```python
from build123d import *

# Parameters (mm, degrees)
BOSS_EXTRUDE1_DEPTH = 40
BOSS_EXTRUDE2_START = -10
SKETCH2_W           = 20
SKETCH2_H           = 50
BOSS_EXTRUDE2_DEPTH = 20
FILLET1_R           = 5
FILLET2_R           = 2
SKETCH3_W           = 45
SKETCH3_H           = 40
BOSS_EXTRUDE3_DEPTH = 5
FILLET3_R           = 5
SKETCH4_R           = 1.55
CUT_EXTRUDE1_DEPTH  = 5
MIRROR4_START       = 60
MIRROR4_OUTLINE_R   = 1.55
MIRROR4_DEPTH       = 5
SKETCH5_W           = 35
SKETCH5_H           = 10
BOSS_EXTRUDE4_DEPTH = 2
FILLET4_R           = 2


# Read off the part's stored shape, not the designer's step: Mirror4
with BuildPart() as part:
    # Sketch1 → Boss-Extrude1 (new body)
    with BuildSketch(Plane(origin=(0, 0, 0), x_dir=(0, 0, -1), z_dir=(1, 0, 0))):
        Polygon((-11.4, 0), (-17.5, 0), (-17.5, 10), (17.5, 10), (17.5, 0), (11.4, 0), (11.4, 2.35), (13.9, 2.35), (13.9, 7.6), (3.6, 7.6), (3.6, 2.35), (6.1, 2.35), (6.1, 0), (-6.1, 0), (-6.1, 2.35), (-3.6, 2.35), (-3.6, 7.6), (-13.9, 7.6), (-13.9, 2.35), (-11.4, 2.35), align=None)
    extrude(amount=BOSS_EXTRUDE1_DEPTH)

    # Sketch2 → Boss-Extrude2 (add)
    with BuildSketch(Plane(origin=(40, 0, 0), x_dir=(0, 0, -1), z_dir=(1, 0, 0)).offset(BOSS_EXTRUDE2_START)):
        with Locations((0, 35)):
            Rectangle(SKETCH2_W, SKETCH2_H)
    extrude(amount=-BOSS_EXTRUDE2_DEPTH)

    # Fillet1
    fillet1_edges = [part.edges().sort_by_distance(p)[0] for p in [
        (10, 35, 10),
        (20, 10, 10),
        (10, 35, -10),
        (10, 10, 0),
        (20, 10, -10),
        (30, 35, 10),
        (30, 10, 0),
        (30, 35, -10),
    ]]
    fillet(fillet1_edges, radius=FILLET1_R)

    # Fillet2
    fillet2_edges = [part.edges().sort_by_distance(p)[0] for p in [
        (20, 10, 17.5),
        (20, 10, -17.5),
    ]]
    fillet(fillet2_edges, radius=FILLET2_R)

    # Sketch3 → Boss-Extrude3 (add)
    with BuildSketch(Plane(origin=(0, 60, 0), x_dir=(1, 0, 0), z_dir=(0, 1, 0))):
        with Locations((20, 0)):
            Rectangle(SKETCH3_W, SKETCH3_H)
    extrude(amount=BOSS_EXTRUDE3_DEPTH)

    # Fillet3
    fillet3_edges = [part.edges().sort_by_distance(p)[0] for p in [
        (20, 60, 10),
        (30, 60, 0),
        (20, 60, -10),
        (10, 60, 0),
        (28.535533906, 60, 8.535533906),
        (28.535533906, 60, -8.535533906),
        (11.464466094, 60, 8.535533906),
        (11.464466094, 60, -8.535533906),
    ]]
    fillet(fillet3_edges, radius=FILLET3_R)

    # Sketch4 → Cut-Extrude1 (cut)
    with BuildSketch(Plane(origin=(0, 65, 0), x_dir=(1, 0, 0), z_dir=(0, 1, 0))):
        with Locations(Location((2.5, 15, 0), (0, 0, 270))):
            Circle(SKETCH4_R)
    extrude(amount=-CUT_EXTRUDE1_DEPTH, mode=Mode.SUBTRACT)

    # Mirror4 outline → Mirror4 (cut)
    with BuildSketch(Plane(origin=(0, 0, 0), x_dir=(1, 0, 0), z_dir=(0, 1, 0)).offset(MIRROR4_START)):
        with Locations((2.5, -15)):
            Circle(MIRROR4_OUTLINE_R)
        with Locations((37.5, 15)):
            Circle(MIRROR4_OUTLINE_R)
        with Locations((37.5, -15)):
            Circle(MIRROR4_OUTLINE_R)
    extrude(amount=MIRROR4_DEPTH, mode=Mode.SUBTRACT)

    # Sketch5 → Boss-Extrude4 (add)
    with BuildSketch(Plane(origin=(40, 0, 0), x_dir=(0, 0, -1), z_dir=(1, 0, 0))):
        with Locations((0, 5)):
            Rectangle(SKETCH5_W, SKETCH5_H)
    extrude(amount=BOSS_EXTRUDE4_DEPTH)

    # Fillet4
    fillet4_edges = [part.edges().sort_by_distance(p)[0] for p in [
        (41, 10, -17.5),
        (41, 10, 17.5),
    ]]
    fillet(fillet4_edges, radius=FILLET4_R)


solid = part.part
```
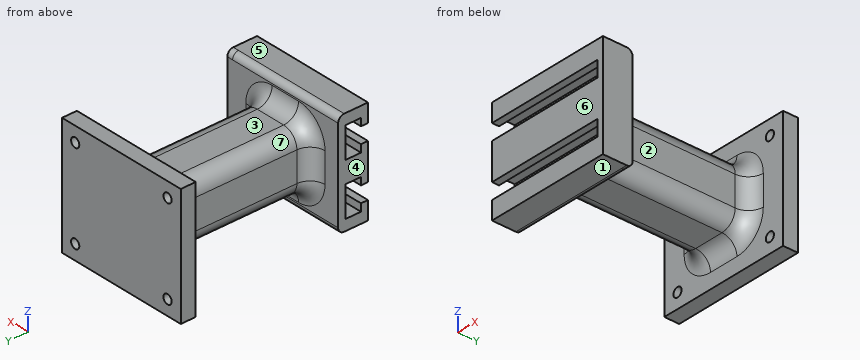
Geometry check sheet. Reference: the model listing, model coordinates, mm. Face numbers are marked on the shaded views. A direction names the side the tool comes from. Give positions to 0.01 mm unless a question says otherwise; leave off trailing zeros. Write each loop counter-clockwise with the first axis right and the second up, starting at its lowest first coordinate (ties: lowest second). Pieces come first, ordered by that corner, then holes. Notation, with made-up numbers: (-22, -30.5) -> (-1, -30.5) arc R18 ccw to (-1, -4.5) -> close; hole circle Ø7 at (-8, -23). An arc over 180 degrees is marked (long way). Use one line per item in the form item = value.
Item 1: Depth check by flat-ended pin: pin 1 Ø0.7 at (x, y) = (27, 1.5) entering from +Z; pin 2 Ø2.5 at (x, z) = (2.5, -15) entering from +Y; pin 3 Ø8 at (y, z) = (38, -2.5) entering from +X; pin 4 Ø5 at (x, z) = (12.5, -10.5) entering from -Y. Enter the tip coordinate at first touch or a pass-through.
Results list:
pin_1 = 17.5
pin_2 = 10
pin_3 = 30
pin_4 = 0
Item 2: Mould release check, pull along Y, two halves, no side actions. Record for the marked faces 5, 6 and 7: released by +Y, released by -Y, zero draft, split by the parting line, or undercut.
Results list:
face_5 = zero draft
face_6 = released by -Y
face_7 = undercut
Item 3: Sectioned sample at A-A on x = 37.5. Count the separate pieces of the cut face and the enclosed holes in it, plus the area to 3 significant figures.
Results list:
separate_pieces = 4
enclosed_holes = 0
area = 384 mm2
Item 4: Sectioned sample at B-B on y = 27.5. Enter the section's corners in (x, z).
Results list:
outline = (10, -5) arc R5 ccw to (15, -10) -> (25, -10) arc R5 ccw to (30, -5) -> (30, 5) arc R5 ccw to (25, 10) -> (15, 10) arc R5 ccw to (10, 5) -> close
Item 5: Access from +Z, -Z, +X, -X, +Y, -Y to the whole of each face (thin tool, end or side, straight path). Record for the marked faces 1, 2, 3 and 4.
Results list:
face_1 = -Z, +X, -X, -Y
face_2 = +Z, -Z, +X
face_3 = +Z, +X, -X
face_4 = +Z, -Z, -X, -Y
Item 6: Sectioned sample at D-D on y = 14. Enter the section's corners in (x, z), plus the area to 3 significant figures.
Results list:
outline = (9.9, -5) arc R5.1 ccw to (15, -10.1) -> (25, -10.1) arc R5.1 ccw to (30.1, -5) -> (30.1, 5) arc R5.1 ccw to (25, 10.1) -> (15, 10.1) arc R5.1 ccw to (9.9, 5) -> close
area = 386 mm2
Item 7: Scan lines: line 1 (X direction, y = 61.4, z = -15); line 2 (Z direction, x = 18.5, y = 7); line 3 (Z direction, x = 37.5, y = 61.35). Record each from-to range of solid material in increasing order.
Results list:
line_1 = -2.5 to 0.95, 4.05 to 35.95, 39.05 to 42.5
line_2 = -17.5 to -13.9, -3.6 to 3.6, 13.9 to 17.5
line_3 = -20 to -16.55, -13.45 to 13.45, 16.55 to 20
